For this review, take the finished solid that the model builds, in its own axes (mm). A direction names the side the tool comes from. Round coordinates to 2 decimals unless told otherwise and drop trailing zeros. Loops run counter-clockwise (first coordinate to the right, second up) from the corner with the lowest first, then second, coordinate; pieces in that order, holes last. Notation, with made-up numbers: (12.25, -4) -> (54.25, -4) arc R18 cw to (54.25, 12) -> close; hole circle Ø2 at (31, 72). An arc over 180 degrees is marked (long way). One line per question, with ' | ' between items. Start each with the question number.
1. For pin 1 Ø2.5 at (x, y) = (69.27, -5) entering from +Z, flat-tipped, find the tip position at first contact; note if it passes through.
2. Draft analysis for pull direction X (two halves, no side actions). For faces 1 (the face through (80.7, -4.55, 2.96)), 2 (the face through (-1, -8, 3)), 3 (the face through (84.27, 0, 3)), state which applies: pulls with the +X half, pulls with the -X half, needs draft (parallel to the pull), parting line crosses it, or undercut.
3. Consider section C-C (z = 2.7). Count the separate pieces of the cut face and the enclosed holes in it, and give its area (3 significant figures).
4. Consider section B-B (x = -79.27). Write out the cut boundary in (y, z), and give its area (3 significant figures).
5. Wall thickness on line 1 along Y through (x, z) = (-79.27, 1.95); line 2 along Y through (x, z) = (-52, 1.95); line 3 along X through (y, z) = (0.25, 1.75): over which ranges is each line inside the solid? List them lowest first.
6. For faces 4 (the face through (-1, 8, 3)), 5 (the face through (-1, -2.5, 3)), list the 3-axis set-ups (+Z, -Z, +X, -X, +Y, -Y) from which the entire face can be reached by the end or side of a thin tool; tool diameter is ignored.
7. Consider section A-A (x = -51.5). Write out the cut boundary in (y, z), and give its area (3 significant figures).
```python
from build123d import *

# Parameters (mm, degrees)
SKETCH_1_W          = 168.54
SKETCH_1_H          = 16
SKETCH_1_R          = 1.5
EXTRUDE_1_DEPTH     = 6
FILLET_1_R          = 2
SKETCH_2_W          = 120
SKETCH_2_H          = 5
CUT_EXTRUDE_1_DEPTH = 6
FILLET_2_R          = 2


with BuildPart() as part:
    # 草图1 → 凸台-拉伸1 (new body)
    with BuildSketch(Plane.XY):
        Rectangle(SKETCH_1_W, SKETCH_1_H)
        with Locations((79.27, 5)):
            Circle(SKETCH_1_R, mode=Mode.SUBTRACT)
        with Locations((69.27, 5)):
            Circle(SKETCH_1_R, mode=Mode.SUBTRACT)
        with Locations((69.27, -5)):
            Circle(SKETCH_1_R, mode=Mode.SUBTRACT)
        with Locations((79.27, -5)):
            Circle(SKETCH_1_R, mode=Mode.SUBTRACT)
        with Locations(Location((-79.27, -5, 0), (0, 0, 180))):
            Circle(SKETCH_1_R, mode=Mode.SUBTRACT)
        with Locations(Location((-69.27, -5, 0), (0, 0, 180))):
            Circle(SKETCH_1_R, mode=Mode.SUBTRACT)
        with Locations(Location((-69.27, 5, 0), (0, 0, 180))):
            Circle(SKETCH_1_R, mode=Mode.SUBTRACT)
        with Locations(Location((-79.27, 5, 0), (0, 0, 180))):
            Circle(SKETCH_1_R, mode=Mode.SUBTRACT)
    extrude(amount=EXTRUDE_1_DEPTH)

    # 圆角1
    fillet_1_edges = [part.edges().sort_by_distance(p)[0] for p in [
        (84.27, -8, 3),
        (-84.27, -8, 3),
        (-84.27, 8, 3),
        (84.27, 8, 3),
    ]]
    fillet(fillet_1_edges, radius=FILLET_1_R)

    # 草图2 → 切除-拉伸1 (cut)
    with BuildSketch(Plane.XY.offset(6)):
        Rectangle(SKETCH_2_W, SKETCH_2_H)
    extrude(amount=-CUT_EXTRUDE_1_DEPTH, mode=Mode.SUBTRACT)

    # 圆角2
    fillet_2_edges = [part.edges().sort_by_distance(p)[0] for p in [
        (60, 2.5, 3),
        (60, -2.5, 3),
        (-60, -2.5, 3),
        (-60, 2.5, 3),
    ]]
    fillet(fillet_2_edges, radius=FILLET_2_R)


solid = part.part
```
Answer block:
1) pin 1: passes through
2) face 1: undercut | face 2: needs draft | face 3: pulls with the +X half
3) separate pieces: 1 | enclosed holes: 9 | area: 2,040 mm2
4) outline: (-8, 0) -> (-6.5, 0) -> (-6.5, 6) -> (-8, 6) -> close; (-3.5, 0) -> (3.5, 0) -> (3.5, 6) -> (-3.5, 6) -> close; (6.5, 0) -> (8, 0) -> (8, 6) -> (6.5, 6) -> close | area: 60.0 mm2
5) line 1: y = -8 to -6.5, -3.5 to 3.5, 6.5 to 8 | line 2: y = -8 to -2.5, 2.5 to 8 | line 3: x = -84.27 to -60, 60 to 84.27
6) face 4: +Z, -Z, +X, -X, +Y | face 5: +Z, -Z
7) outline: (-8, 0) -> (-2.5, 0) -> (-2.5, 6) -> (-8, 6) -> close; (2.5, 0) -> (8, 0) -> (8, 6) -> (2.5, 6) -> close | area: 66.0 mm2
